from build123d import *

# Parameters (mm, degrees)
SKETCH1_W           = 126
SKETCH1_H           = 60
SKETCH1_R           = 1.5
BOSS_EXTRUDE1_DEPTH = 1.5
SKETCH2_W           = 100
SKETCH2_H           = 50
BOSS_EXTRUDE2_DEPTH = 2
SKETCH3_W           = 106
SKETCH3_H           = 60
BOSS_EXTRUDE3_DEPTH = 1
FILLET1_R           = 5
SKETCH4_W           = 86
SKETCH4_H           = 54
CUT_EXTRUDE1_DEPTH  = 0.01
SKETCH6_W           = 18
SKETCH6_H           = 18
CUT_EXTRUDE2_DEPTH  = 1.5
SKETCH7_W           = 20
SKETCH7_H           = 2
SKETCH7_W_2         = 15
SKETCH7_W_3         = 25
BOSS_EXTRUDE4_DEPTH = 9
SKETCH8_W           = 3
SKETCH8_H           = 9
CUT_EXTRUDE3_DEPTH  = 2
SKETCH9_W           = 5
SKETCH9_H           = 6
BOSS_EXTRUDE5_DEPTH = 4
SKETCH10_R          = 1.5
CUT_EXTRUDE4_DEPTH  = 1
FILLET2_R           = 1


with BuildPart() as part:
    # Sketch1 → Boss-Extrude1 (new body)
    with BuildSketch(Plane(origin=(0, 0, 0), x_dir=(1, 0, 0), z_dir=(0, 1, 0))):
        Rectangle(SKETCH1_W, SKETCH1_H)
        with Locations(Location((-59, 26, 0), (0, 0, 270))):
            Circle(SKETCH1_R, mode=Mode.SUBTRACT)
        with Locations(Location((-59, -26, 0), (0, 0, 90))):
            Circle(SKETCH1_R, mode=Mode.SUBTRACT)
        with Locations(Location((59, -26, 0), (0, 0, 270))):
            Circle(SKETCH1_R, mode=Mode.SUBTRACT)
        with Locations(Location((59, 26, 0), (0, 0, 90))):
            Circle(SKETCH1_R, mode=Mode.SUBTRACT)
    extrude(amount=BOSS_EXTRUDE1_DEPTH)

    # Sketch2 → Boss-Extrude2 (add)
    with BuildSketch(Plane(origin=(0, 1.5, 0), x_dir=(1, 0, 0), z_dir=(0, 1, 0))):
        Rectangle(SKETCH2_W, SKETCH2_H)
    extrude(amount=BOSS_EXTRUDE2_DEPTH)

    # Sketch3 → Boss-Extrude3 (add)
    with BuildSketch(Plane(origin=(0, 3.5, 0), x_dir=(1, 0, 0), z_dir=(0, 1, 0))):
        Rectangle(SKETCH3_W, SKETCH3_H)
    extrude(amount=BOSS_EXTRUDE3_DEPTH)

    # Fillet1
    fillet1_edges = [part.edges().sort_by_distance(p)[0] for p in [
        (53, 4, 30),
        (53, 4, -30),
        (-53, 4, -30),
        (-53, 4, 30),
    ]]
    fillet(fillet1_edges, radius=FILLET1_R)

    # Sketch4 → Cut-Extrude1 (cut)
    with BuildSketch(Plane(origin=(0, 4.5, 0), x_dir=(1, 0, 0), z_dir=(0, 1, 0))):
        Rectangle(SKETCH4_W, SKETCH4_H)
    extrude(amount=-CUT_EXTRUDE1_DEPTH, mode=Mode.SUBTRACT)

    # Sketch6 → Cut-Extrude2 (cut)
    with BuildSketch(Plane.XZ):
        with Locations((43, 13)):
            Rectangle(SKETCH6_W, SKETCH6_H)
    extrude(amount=-CUT_EXTRUDE2_DEPTH, mode=Mode.SUBTRACT)

    # Sketch7 → Boss-Extrude4 (add)
    with BuildSketch(Plane.XZ):
        with Locations((13, 24)):
            Rectangle(SKETCH7_W, SKETCH7_H)
        with Locations((-6.5, 24)):
            Rectangle(SKETCH7_W_2, SKETCH7_H)
        with Locations((20.5, -24)):
            Rectangle(SKETCH7_W_3, SKETCH7_H)
        with Locations((-4, -24)):
            Rectangle(SKETCH7_W, SKETCH7_H)
    extrude(amount=BOSS_EXTRUDE4_DEPTH)

    # Sketch8 → Cut-Extrude3 (cut)
    with BuildSketch(Plane(origin=(0, 0, -25), x_dir=(-1, 0, 0), z_dir=(0, 0, -1))):
        with Locations((-31.5, -4.5)):
            Rectangle(SKETCH8_W, SKETCH8_H)
    extrude(amount=-CUT_EXTRUDE3_DEPTH, mode=Mode.SUBTRACT)

    # Sketch9 → Boss-Extrude5 (add)
    with BuildSketch(Plane.XZ):
        with Locations((60.5, 0)):
            Rectangle(SKETCH9_W, SKETCH9_H)
    extrude(amount=BOSS_EXTRUDE5_DEPTH)

    # Sketch10 → Cut-Extrude4 (cut)
    with BuildSketch(Plane(origin=(63, 0, 0), x_dir=(0, 0, -1), z_dir=(1, 0, 0))):
        with Locations((0, -1.469545864)):
            Circle(SKETCH10_R)
    extrude(amount=-CUT_EXTRUDE4_DEPTH, mode=Mode.SUBTRACT)

    # Fillet2
    fillet2_edges = [part.edges().sort_by_distance(p)[0] for p in [
        (60.5, -4, 3),
        (60.5, -4, -3),
    ]]
    fillet(fillet2_edges, radius=FILLET2_R)


solid = part.part
Work out the finished part from the listing and answer in its coordinate system (mm). A direction names the side the tool comes from. Round coordinates to 2 decimals unless told otherwise and drop trailing zeros. Write each loop counter-clockwise with the first axis right and the second up, starting at its lowest first coordinate (ties: lowest second). Pieces come first, ordered by that corner, then holes.
1) A tool of negligible diameter and unlimited length cuts with its end or side. For faces 4 (the cylindrical face through (-52, 4, -28)), 5 (the flat face through (-4, -4, -23)), 6 (the flat face through (-4, -4, -25)), from which of +Z, -Z, +X, -X, +Y, -Y can it reach the whole face along a straight path? Write none if from no direction.
2) The mould has two halves that part along Z. Classify faces 1 (the flat face through (19, -4, -25)), 2 (the flat face through (-1, 1.5, 26)), 3 (the flat face through (42, 1.5, 13)): pulls with the +Z half, pulls with the -Z half, needs draft (parallel to the pull), parting line crosses it, or undercut.
3) A cutting plane is placed at A-A (y = -5.75). Give the vertices of the cut face in (x, z), plus the area to 3 significant figures.
4) Given pin 1 Ø17.5 at (x, z) = (46, 13.5) entering from -Y; pin 2 Ø2 at (x, z) = (60.5, 0) entering from -Y; pin 3 Ø0.9 at (x, y) = (61.5, -1.5) entering from -Z, each flat-ended and moving along its own axis, determine where each tip first touches the part or whether it passes through.
5) Straight lines are drawn through the part: line 1 (X direction, y = 1.2, z = 26); line 2 (Z direction, x = 41.5, y = 1.25); line 3 (Z direction, x = 12, y = -3.5). For each, find the intervals that lie inside material, in ascending order.
6) A cutting plane is placed at B-B (x = -59). Give the vertices of the cut face in (y, z), plus the area to 3 significant figures.
Completed:
1. face 4: -Z, -X, +Y
1. face 5: +X, -X, -Y
1. face 6: -Z, +X, -X, -Y
2. face 1: pulls with the -Z half
2. face 2: needs draft
2. face 3: undercut
3. outline: (-14, -25) - (6, -25) - (6, -23) - (-14, -23) - close; (-14, 23) - (1, 23) - (1, 25) - (-14, 25) - close; (3, 23) - (23, 23) - (23, 25) - (3, 25) - close; (8, -25) - (30, -25) - (30, -23) - (8, -23) - close
3. area: 154 mm2
4. pin 1: stops at y = 0
4. pin 2: stops at y = -4
4. pin 3: stops at z = -3
5. line 1: x = -63 to -60.5, -57.5 to 57.5, 60.5 to 63
5. line 2: z = -30 to 4, 22 to 30
5. line 3: z = -25 to -23, 23 to 25
6. outline: (0, -30) - (1.5, -30) - (1.5, -27.5) - (0, -27.5) - close; (0, -24.5) - (1.5, -24.5) - (1.5, 24.5) - (0, 24.5) - close; (0, 27.5) - (1.5, 27.5) - (1.5, 30) - (0, 30) - close
6. area: 81.0 mm2
